```python
from build123d import *

# Parameters (mm, degrees)
BOSS_EXTRUDE1_DEPTH      = 0.01
BOSS_EXTRUDE1_DEPTH_BACK = 5
SKETCH5_R                = 2.45
SKETCH5_R_2              = 1.5
BOSS_EXTRUDE2_DEPTH      = 5


with BuildPart() as part:
    # Sketch1 → Boss-Extrude1 (new, two sides: drawn at the far end of the back side and taken through both)
    with BuildSketch(Plane(origin=(0.212370974, 88.261171587, 0), x_dir=(0.9999971051966906, -0.0024061583985667905, 0), z_dir=(0.0024061583985667905, 0.9999971051966906, 2.2915916530952404e-15)).offset(-BOSS_EXTRUDE1_DEPTH_BACK)):
        with BuildLine():
            add(Edge.make_bspline(
                [(62.098697441, -271.553297735), (62.098697441, -271.390083561), (62.082868678, -271.227746225), (62.018744893, -270.904868209), (61.970774481, -270.747219765), (61.846181156, -270.44635233), (61.768554488, -270.300830702), (61.586127547, -270.027822449), (61.482834878, -269.902064788), (61.252588694, -269.671493322), (61.124154836, -269.565937636), (60.85291301, -269.384527638), (60.709509325, -269.307646832), (60.406882072, -269.181865969), (60.248191704, -269.13364771), (59.928627436, -269.06981324), (59.765989129, -269.053431748), (59.435435386, -269.053165346), (59.272896926, -269.069262853), (58.953071086, -269.132607362), (58.794102275, -269.180650645), (58.491413646, -269.30591032), (58.347818746, -269.382585434), (58.075961384, -269.563834415), (57.947444391, -269.669183663), (57.601723344, -270.014407111), (57.415265036, -270.29289619), (57.16528984, -270.894119026), (57.098697441, -271.222630203), (57.098697441, -271.553297735)],
                knots=[0, 0, 0, 0, 0.0625, 0.0625, 0.125, 0.125, 0.1875, 0.1875, 0.25, 0.25, 0.3125, 0.3125, 0.375, 0.375, 0.4375, 0.4375, 0.5, 0.5, 0.5625, 0.5625, 0.625, 0.625, 0.6875, 0.6875, 0.75, 0.75, 0.875, 0.875, 1, 1, 1, 1], degree=3))
            Line((57.098697441, -271.553297735), (57.098697441, -288.700730466))
            add(Edge.make_bspline(
                [(57.098697441, -291.553297735), (57.098716176, -291.500037735), (57.098733901, -291.446736965), (57.098944046, -290.775972975), (57.098997483, -290.169015827), (57.098876087, -289.279212217), (57.098803426, -288.988725401), (57.098697441, -288.700730466)],
                knots=[0.466050383, 0.466050383, 0.466050383, 0.466050383, 0.46875, 0.46875, 0.5, 0.5, 0.515336825, 0.515336825, 0.515336825, 0.515336825], degree=3))
            add(Edge.make_bspline(
                [(59.695767456, -294.051424481), (59.664952853, -294.052615647), (59.634064807, -294.053239292), (59.43288412, -294.053593818), (59.260500841, -294.036058258), (58.929915117, -293.968086951), (58.767684875, -293.9170646), (58.460210959, -293.785297782), (58.316149887, -293.70550705), (58.0458038, -293.51937365), (57.92043612, -293.413227178), (57.583512234, -293.067438733), (57.404616617, -292.79348169), (57.223603479, -292.349815403), (57.176716166, -292.193718571), (57.11440851, -291.876470519), (57.098697441, -291.715881831), (57.098697441, -291.553297735)],
                knots=[0.488631618, 0.488631618, 0.488631618, 0.488631618, 0.5, 0.5, 0.5625, 0.5625, 0.625, 0.625, 0.6875, 0.6875, 0.75, 0.75, 0.875, 0.875, 0.9375, 0.9375, 1, 1, 1, 1], degree=3))
            Line((59.695767456, -294.051424481), (59.695767456, -275.672418356))
            Line((59.695767456, -275.672418356), (62.098697441, -271.553297735))
        make_face()
    extrude(amount=BOSS_EXTRUDE1_DEPTH + BOSS_EXTRUDE1_DEPTH_BACK)

    # Sketch5 → Boss-Extrude2 (add)
    # profile 1 of 2: a face of its own
    with BuildSketch(Plane(origin=(0.212370974, 88.261171587, 0), x_dir=(0.9999971051966906, -0.0024061583985667905, 0), z_dir=(0.0024061583985667905, 0.9999971051966906, 2.2915916530952404e-15))):
        with Locations(Location((58.382444571, -274.369066811, 0), (0, 0, 12.765246623))):
            Circle(SKETCH5_R)
        with Locations(Location((58.382444571, -274.369066811, 0), (0, 0, 211.148291833))):
            Circle(SKETCH5_R_2, mode=Mode.SUBTRACT)
    # profile 2 of 2: a face of its own
    with BuildSketch(Plane(origin=(0.212370974, 88.261171587, 0), x_dir=(0.9999971051966906, -0.0024061583985667905, 0), z_dir=(0.0024061583985667905, 0.9999971051966906, 2.2915916530952404e-15))):
        with Locations((58.382444571, -288.73753777)):
            Circle(SKETCH5_R)
        with Locations((58.382444571, -288.73753777)):
            Circle(SKETCH5_R_2, mode=Mode.SUBTRACT)
    extrude(amount=BOSS_EXTRUDE2_DEPTH)


solid = part.part
```
Read the model definition and answer for the solid it produces. Units are mm, in the model's axes. Coordinates: 2 decimals unless noted, no trailing zeros. Write each loop counter-clockwise with the first axis right and the second up, starting at its lowest first coordinate (ties: lowest second). Pieces come first, ordered by that corner, then holes. Notation, with made-up numbers: (43.25, -35.75) - (87.25, -35.75) arc R11 cw to (87.25, -17.75) - close; hole circle Ø5 at (27.5, 22.25). An arc over 180 degrees is marked (long way). Answer as a JSON object with one key per item and string values. Group by question number.
1. A cutting plane is placed at C-C (z = 287.5). Determine the outline of the cut face in (x, y), plus the area to 3 significant figures.
2. A cutting plane is placed at B-B (y = 92). Give the number of separate pieces and of enclosed holes in the cut face, plus the area to 3 significant figures.
3. Consider L1, parallel to Z at x = 59.25, y = 92.5; L2, parallel to Z at x = 58.25, y = 90.5; L3, parallel to X at y = 84, z = 280.25. Determine where each line is inside the solid, lowest interval first. Write a range as [from, to].
4. The mould has two halves that part along Z. Classify faces 1 (the cylindrical face through (58.61, 90.59, 276.82)), 2 (the cylindrical face through (59.918, 90.583, 286.672)): +Z half, -Z half, draft (parallel to the pull), parting line (faces both ways), or undercut.
5. Each of these flat-tipped pins is pushed along its axis until it touches: P1, Ø1, axis at y = 86.5, z = 283.5, coming from the -X side; P2, Ø1, axis at x = 58.5, z = 289, coming from the -Y side; P3, Ø1.5, axis at x = 61, z = 275.5, coming from the +Y side. Where does it stop, or does it pass through?
6. A cutting plane is placed at A-A (z = 283.25). Determine the outline of the cut face in (x, y).
Worked out:
{
 "1": {"outline": "(56.48, 88.13) - (57.31, 88.12) - (57.3, 83.12) - (59.9, 83.12) - (59.91, 88.12) - (60.71, 88.12) - (60.72, 93.12) - (59.45, 93.12) - (59.44, 88.13) - (57.75, 88.13) - (57.76, 93.12) - (56.49, 93.13) - close", "area": "25.7 mm²"},
 "2": {"separate pieces": "2", "enclosed holes": "2", "area": "23.6 mm²"},
 "3": {"L1": "z = [272.01, 273.01], [275.72, 276.73], [286.37, 287.38], [290.09, 291.1]", "L2": "z = [271.94, 272.91], [275.83, 276.79], [286.31, 287.28], [290.2, 291.16]", "L3": "x = [57.3, 59.9]"},
 "4": {"face 1": "undercut", "face 2": "undercut"},
 "5": {"P1": "stops at x = 57.31", "P2": "stops at y = 83.12", "P3": "stops at y = 93.12"},
 "6": {"outline": "(57.3, 83.12) - (59.9, 83.12) - (59.91, 88.13) - (57.31, 88.13) - close"}
}
